CAD build for the part. Positions are in the model's coordinates, mm. A direction names the side the tool comes from. Give positions to 0.01 mm unless a question says otherwise; leave off trailing zeros. Write each loop counter-clockwise with the first axis right and the second up, starting at its lowest first coordinate (ties: lowest second). Pieces come first, ordered by that corner, then holes. Notation, with made-up numbers: (75, -30) - (94, -30) arc R20 ccw to (94, -7) - close; hole circle Ø4 at (1.25, 53). An arc over 180 degrees is marked (long way). Answer as a JSON object with one key per item and string values.
from build123d import *

# Parameters (mm, degrees)
F1_DEPTH = 45
F3_D     = 5
F5_D     = 5
F7_D     = 5
F9_D     = 5
F10_R    = 7.62
F11_R    = 5.08


with BuildPart() as f1:
    # F0 (on Front) → F1 (new body)
    with BuildSketch(Plane.XZ):
        Polygon((50, 20), (20, 20), (10, 20), (0, 10), (-10, 20), (-20, 20), (-50, 20), (-50, 0), (-50, -10), (50, -10), (50, 0), align=None)
    extrude(amount=F1_DEPTH)

    # F3 (through all)
    with Locations(Plane.XY.offset(20)):
        with Locations((35, -35)):
            Hole(F3_D / 2)

    # F5 (through all)
    with Locations(Plane.XY.offset(20)):
        with Locations((35, -10)):
            Hole(F5_D / 2)

    # F7 (through all)
    with Locations(Plane.XY.offset(20)):
        with Locations((-35, -10)):
            Hole(F7_D / 2)

    # F9 (through all)
    with Locations(Plane.XY.offset(20)):
        with Locations((-35, -35)):
            Hole(F9_D / 2)

    # F10
    f10_edges = [f1.edges().sort_by_distance(p)[0] for p in [
        (10, -22.5, 20),
        (-10, -22.5, 20),
    ]]
    fillet(f10_edges, radius=F10_R)

    # F11
    f11_edges = [f1.edges().sort_by_distance(p)[0] for p in [
        (-31.578154, -45, 20),
        (31.578154, -45, 20),
        (31.578154, 0, 20),
        (-31.578154, 0, 20),
    ]]
    fillet(f11_edges, radius=F11_R)


solid = f1.part
Item 1: Which spindle directions (+Z, -Z, +X, -X, +Y, -Y) get a long thin tool onto all of the face, cutting with end or side? Do faces 1 (the cylindrical face through (-10.202, -22.744, 19.404)), 2 (the cylindrical face through (-4.51, -43.55, 12.35)), 3 (the cylindrical face through (-37.31, -10.96, 4.79)), 4 (the cylindrical face through (-4.51, -1.45, 12.35)). Say none if no direction does.
Entries:
{"face 1": "+Z, +Y, -Y", "face 2": "+Z, -Y", "face 3": "+Z, -Z", "face 4": "+Z, +Y"}
Item 2: Cut at D-D (y = -24.5). Give the cut face in (x, z), and give its area (3 significant figures).
Entries:
{"outline": "(-50, -10) - (50, -10) - (50, 20) - (13.16, 20) arc R7.62 ccw to (7.77, 17.77) - (0, 10) - (-7.77, 17.77) arc R7.62 ccw to (-13.16, 20) - (-50, 20) - close", "area": "2,900 mm2"}
Item 3: Cut at C-C (z = -4.5). Give the cut face in (x, y).
Entries:
{"outline": "(-50, -45) - (50, -45) - (50, 0) - (-50, 0) - close; hole circle Ø5 at (-35, -35); hole circle Ø5 at (-35, -10); hole circle Ø5 at (35, -35); hole circle Ø5 at (35, -10)"}
Item 4: Probe line 1 (Y direction, x = 35, z = -2); line 2 (X direction, y = -10.5, z = 14); line 3 (Z direction, x = -19, y = -40). List the from-to ranges inside material, lowest first. Write a range as from..to.
Entries:
{"line 1": "-45..-37.5, -32.5..-12.5, -7.5..0", "line 2": "-50..-37.45, -32.55..-4, 4..32.55, 37.45..50", "line 3": "-10..20"}
Item 5: Cut at A-A (y = -33.5). Give the cut face in (x, z), and give its area (3 significant figures).
Entries:
{"outline": "(-50, -10) - (-37, -10) - (-37, 20) - (-50, 20) - close; (-33, -10) - (33, -10) - (33, 20) - (13.16, 20) arc R7.62 ccw to (7.77, 17.77) - (0, 10) - (-7.77, 17.77) arc R7.62 ccw to (-13.16, 20) - (-33, 20) - close; (37, -10) - (50, -10) - (50, 20) - (37, 20) - close", "area": "2,660 mm2"}
Item 6: Flat gauge pins, fed straight in: P1, Ø8, axis at x = -35, y = -35, coming from the -Z side; P2, Ø1.5, axis at x = -5, z = 11, coming from the -Y side; P3, Ø2, axis at x = -1, y = -24, coming from the +Z side. Where does each tip first touch, or does it go through?
Entries:
{"P1": "z = -10", "P2": "y = -44.77", "P3": "z = 12"}
Item 7: Mould opens along X. For faces 5 (the cylindrical face through (31.32, -1.528, 18.551)), 6 (the cylindrical face through (-37.385, -34.249, 4.79)), 7 (the flat face through (50, -22, 5)) say: +X half, -X half, draft (parallel to the pull), parting line (faces both ways), or undercut.
Entries:
{"face 5": "draft", "face 6": "undercut", "face 7": "+X half"}
Item 8: Cut at B-B (x = 35). Give the cut face in (y, z), and give its area (3 significant figures).
Entries:
{"outline": "(-45, -10) - (-37.5, -10) - (-37.5, 20) - (-39.92, 20) arc R5.08 ccw to (-45, 14.92) - close; (-32.5, -10) - (-12.5, -10) - (-12.5, 20) - (-32.5, 20) - close; (-7.5, -10) - (0, -10) - (0, 14.92) arc R5.08 ccw to (-5.08, 20) - (-7.5, 20) - close", "area": "1,040 mm2"}
